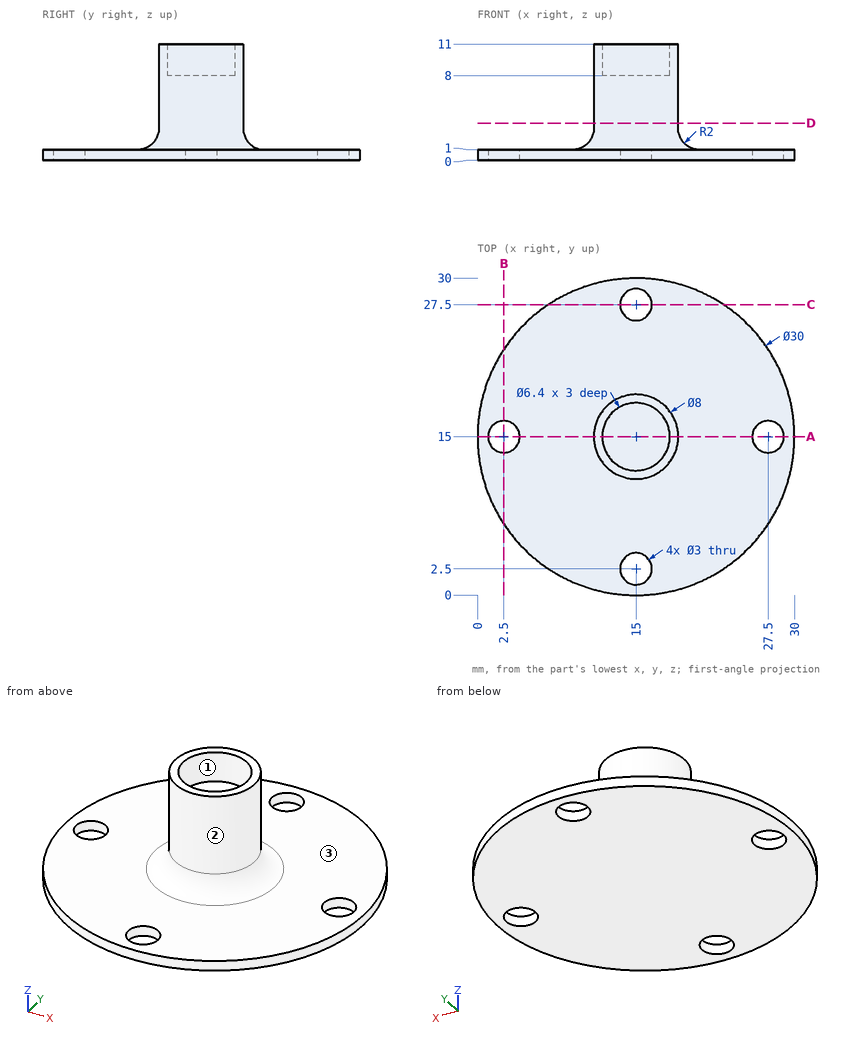
Check sheet for the drawn part. Datum: minimum x, y, z corner. Units: mm. Round coordinates to 2 decimals unless told otherwise and drop trailing zeros. Order: outer loops, then holes, each group sorted by start corner. A loop starts at its lowest first (then second) coordinate and runs counter-clockwise, first axis right, second up. Notation, with made-up numbers: (-15, 11) -> (17, 11) arc R22 ccw to (17, 43) -> close; hole circle Ø8 at (38.25, 34.25). An arc over 180 degrees is marked (long way). Put each result on its own line as item: value. Start each with the question number.
(1) Draft check along X on the marked faces 1, 2 and 3. Enter one of: +X half, -X half, draft (parallel to the pull), parting line (faces both ways), or undercut.
(2) Section check B-B (x = 2.5). Enter the section's corners in (y, z), then the cut area to 3 significant figures.
(3) Section check A-A (y = 15). Enter the section's corners in (x, z), then the cut area to 3 significant figures.
(4) Section check D-D (z = 3.5). Enter the section's corners in (x, y).
(5) Depth check by flat-ended pin: pin 1 Ø6 at (x, z) = (12.5, 2.5) entering from -Y; pin 2 Ø1 at (x, z) = (12.5, 3) entering from +Y; pin 3 Ø2.5 at (x, y) = (27.5, 15) entering from -Z; pin 4 Ø1 at (y, z) = (16.5, 8) entering from +X. Enter the tip coordinate at first touch or a pass-through.
(6) Material ranges on line 1 along Y through (x, z) = (15, 0.5); line 2 along Z through (x, y) = (3, 16.75); line 3 along Y through (x, z) = (27.5, 0.75), recorded low to high.
Completed:
1. face 1: undercut
1. face 2: parting line
1. face 3: draft
2. outline: (6.71, 0) -> (13.5, 0) -> (13.5, 1) -> (6.71, 1) -> close; (16.5, 0) -> (23.29, 0) -> (23.29, 1) -> (16.5, 1) -> close
2. area: 13.6 mm2
3. outline: (0, 0) -> (1, 0) -> (1, 1) -> (0, 1) -> close; (4, 0) -> (26, 0) -> (26, 1) -> (21, 1) arc R2 cw to (19, 3) -> (19, 11) -> (18.2, 11) -> (18.2, 8) -> (11.8, 8) -> (11.8, 11) -> (11, 11) -> (11, 3) arc R2 cw to (9, 1) -> (4, 1) -> close; (29, 0) -> (30, 0) -> (30, 1) -> (29, 1) -> close
3. area: 86.5 mm2
4. outline: circle Ø8 at (15, 15)
5. pin 1: stops at y = 0
5. pin 2: stops at y = 18.46
5. pin 3: passes through
5. pin 4: stops at x = 18.87
6. line 1: y = 0 to 1, 4 to 26, 29 to 30
6. line 2: z = 0 to 1
6. line 3: y = 6.71 to 13.5, 16.5 to 23.29
